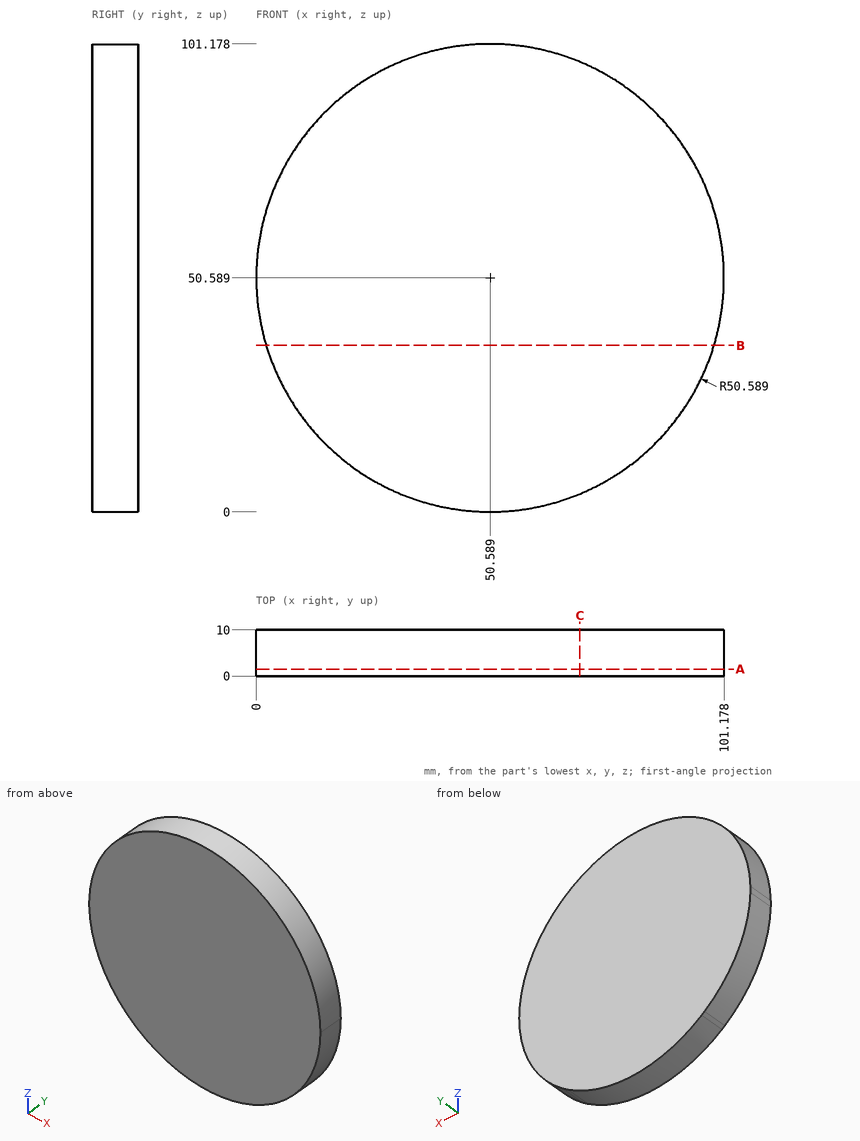
The figure shows three views and two pictorial views of one solid part (mm, origin at its lowest corner). Answer the questions. Coordinates: 2 decimals unless noted, no trailing zeros. Loops run counter-clockwise (first coordinate to the right, second up) from the corner with the lowest first, then second, coordinate; pieces in that order, holes last. Notation, with made-up numbers: (20, -25) - (60, -25) arc R29 ccw to (60, -5) - close; hole circle Ø2 at (67.5, -25.5). An arc over 180 degrees is marked (long way). Use a Markdown table: item, result. Add a question column.
1) The part is cut by section A-A, the plane y = 1.5. Give the vertices of the cut face in (x, z) (1 decimal).
2) The part is cut by section C-C, the plane x = 70. Give the vertices of the cut face in (y, z) (1 decimal).
3) Find the intervals of material crossed by line 1 (X direction, y = 4, z = 79) (1 decimal); line 2 (Z direction, x = 81, y = 2.5) (1 decimal); line 3 (X direction, y = 6.5, z = 58) (1 decimal), in increasing order.
4) The part is cut by section B-B, the plane z = 36. Give the vertices of the cut face in (x, y).
5) Given pin 1 (1 mm diameter, centred on y = 7, z = 48.5, fed in from +X), flat-ended and moving along its own axis, determine where the tip first touches the part or whether it passes through.
Here are the results:
| question | item | result |
|---|---|---|
| 1 | outline | circle Ø101.2 at (50.6, 50.6) |
| 2 | outline | (0, 3.9) - (10, 3.9) - (10, 97.3) - (0, 97.3) - close |
| 3 | line 1 | x = 8.7 to 92.4 |
| 3 | line 2 | z = 10.2 to 91 |
| 3 | line 3 | x = 0.5 to 100.6 |
| 4 | outline | (2.15, 0) - (99.03, 0) - (99.03, 10) - (2.15, 10) - close |
| 5 | pin 1 | stops at x = 101.15 |
